Job drawing, mm, ordinate dimensions from the low corner. One solid piece. A direction names the side the tool comes from. Give positions to 0.01 mm unless a question says otherwise; leave off trailing zeros. Loops run counter-clockwise (first coordinate to the right, second up) from the corner with the lowest first, then second, coordinate; pieces in that order, holes last. Notation, with made-up numbers: M -20,3 L 24,3 A5 cw 24,11 Z; hole C -29,18.25 d8. An arc over 180 degrees is marked long. Put each result on its own line as item: value.
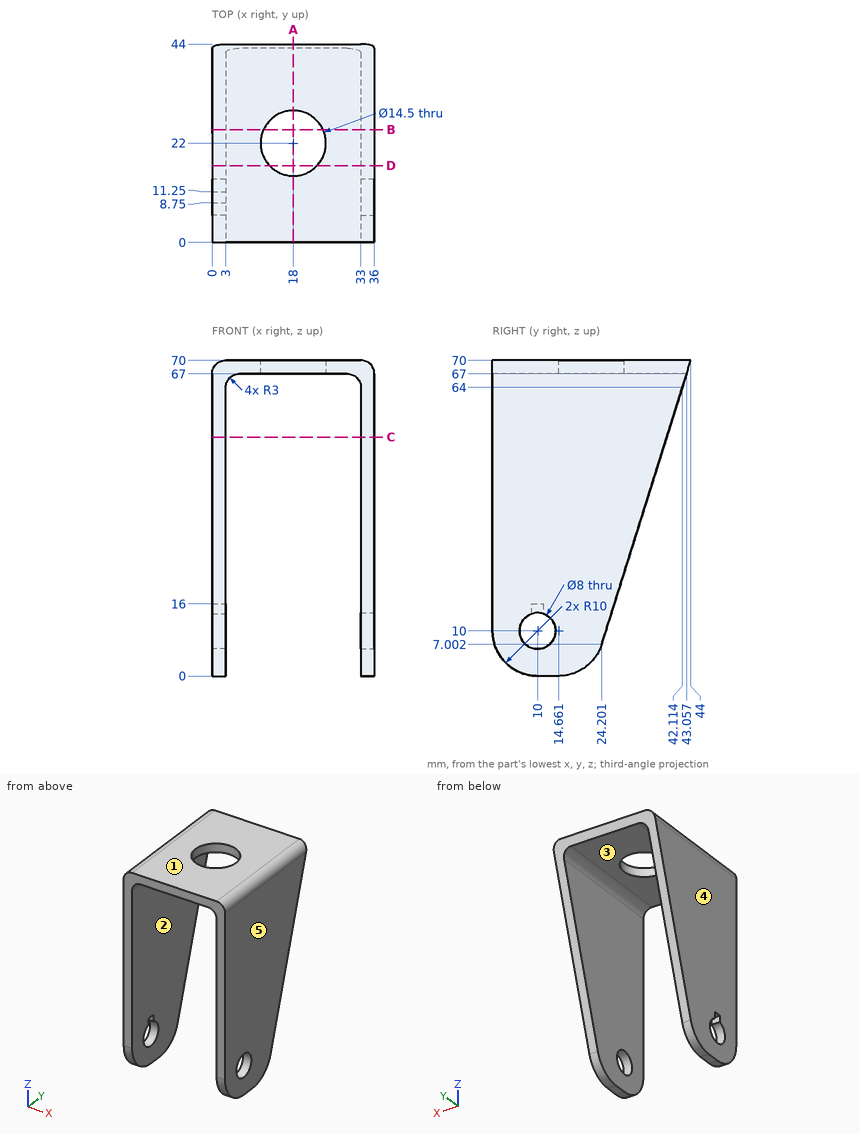
Q1. Mould opens along X. For the marked faces 3, 4 and 5 say: pulls with the +X half, pulls with the -X half, needs draft (parallel to the pull), parting line crosses it, or undercut.
Here are the results:
face 3: undercut
face 4: pulls with the -X half
face 5: pulls with the +X half
Q2. Tool access for the marked faces 1 and 2: list every direction of +Z, -Z, +X, -X, +Y, -Y with a clear straight run to the whole face (end or side of a thin tool).
Here are the results:
face 1: +Z, +X, -X, +Y, -Y
face 2: -Z, +Y, -Y
Q3. Slice it at D-D (y = 17). List the corners of the cut face in (x, z), and give its area (3 significant figures).
Here are the results:
outline: M 0,0.28 L 3,0.28 L 3,64 A3 cw 6,67 L 12.75,67 L 12.75,70 L 3,70 A3 ccw 0,67 Z; M 23.25,67 L 30,67 A3 cw 33,64 L 33,0.28 L 36,0.28 L 36,67 A3 ccw 33,70 L 23.25,70 Z
area: 477 mm²
Q4. Slice it at A-A (x = 18). List the corners of the cut face in (y, z).
Here are the results:
outline: M 0,67 L 14.75,67 L 14.75,70 L 0,70 Z; M 29.25,67 L 43.06,67 L 44,70 L 29.25,70 Z
Q5. Drop flat-ended pins along their axis: pin 1 Ø12 at (x, y) = (12, 19.5) entering from -Z; pin 2 Ø1.1 at (x, z) = (2, 15) entering from +Y. Give the stop position or say it passes through.
Here are the results:
pin 1: z = 67
pin 2: y = 26.89
Q6. Slice it at B-B (y = 25). List the corners of the cut face in (x, z) (1 decimal), and give its area (3 significant figures).
Here are the results:
outline: M 0,9.5 L 3,9.5 L 3,64 A3 cw 6,67 L 11.4,67 L 11.4,70 L 3,70 A3 ccw 0,67 Z; M 24.6,67 L 30,67 A3 cw 33,64 L 33,9.5 L 36,9.5 L 36,67 A3 ccw 33,70 L 24.6,70 Z
area: 413 mm²
Q7. Slice it at C-C (z = 53). List the corners of the cut face in (x, y).
Here are the results:
outline: M 0,0 L 3,0 L 3,38.66 L 0,38.66 Z; M 33,0 L 36,0 L 36,38.66 L 33,38.66 Z
Q8. Probe line 1 (X direction, y = 17.5, z = 36); line 2 (Z direction, x = 8, y = 42); line 3 (Z direction, x = 34, y = 10). List the from-to ranges inside material, lowest first. Write a range as from..to.
Here are the results:
line 1: 0..3, 33..36
line 2: 67..70
line 3: 0..6, 14..69.83
